Verification items for this drawing (mm, ordinates from the low corner). Round coordinates to 2 decimals unless told otherwise and drop trailing zeros. Loops run counter-clockwise (first coordinate to the right, second up) from the corner with the lowest first, then second, coordinate; pieces in that order, holes last. Notation, with made-up numbers: M 9.25,1 L 29.25,1 A25 ccw 29.25,34 Z; hole C 21,81 d4. An arc over 180 degrees is marked long. Write item = value, one per line. Start each with the question number.
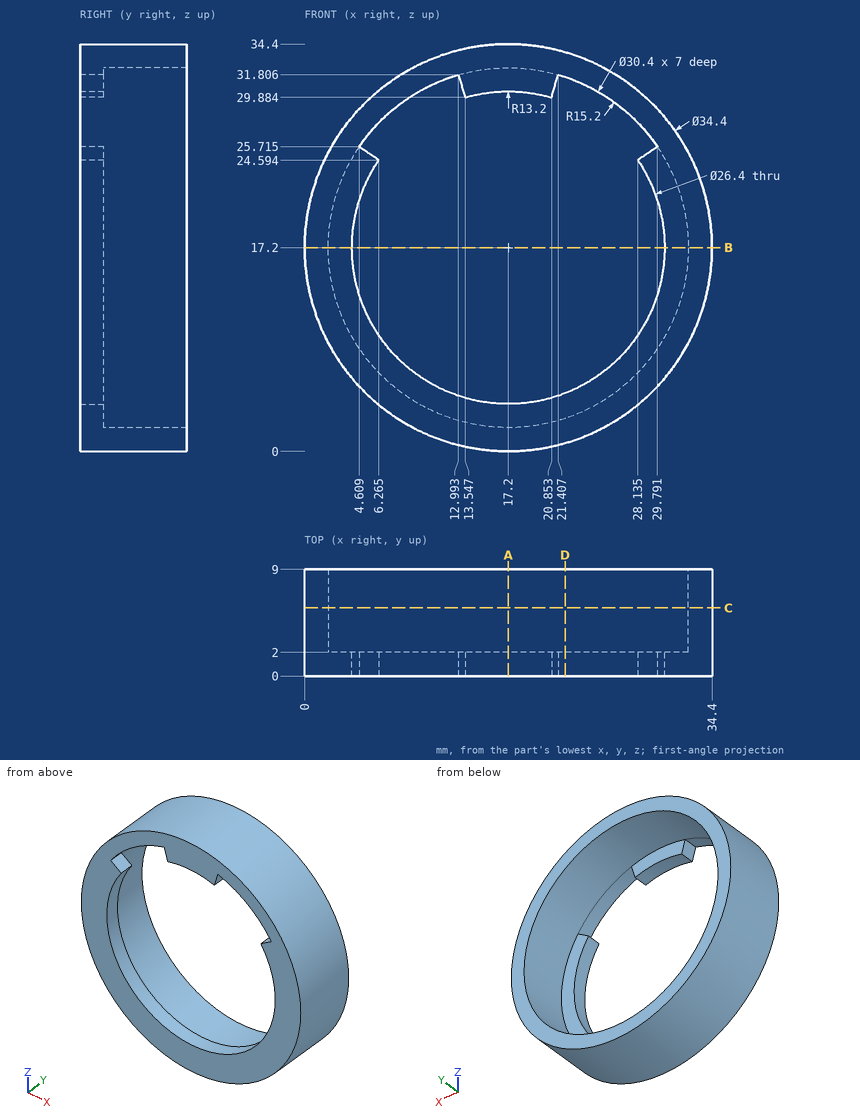
1. Gauge pin test, flat ends, axial feed: P1, Ø18, axis at x = 17.2, z = 17.2, coming from the +Y side; P2, Ø0.8, axis at x = 16, z = 31, coming from the +Y side; P3, Ø3, axis at x = 29.5, z = 12.5, coming from the -Y side; P4, Ø5, axis at y = 3.5, z = 4, coming from the +X side. Record the tip position at first contact, or that the pin passes through.
2. Thickness scan on line 1 (X direction, y = 7, z = 17.2); line 2 (Z direction, x = 17.2, y = 1.1). Record the ranges inside material, lowest first.
3. Section check C-C, the plane y = 5.75. Enter the section's corners in (x, z).
4. Section check A-A, the plane x = 17.2. Enter the section's corners in (y, z).
5. Section check D-D, the plane x = 22. Enter the section's corners in (y, z).
6. Section check B-B, the plane z = 17.2. Enter the section's corners in (x, y).
Computed values:
q1.P1 = through
q1.P2 = 2
q1.P3 = 0
q1.P4 = 30.67
q2.line_1 = 0 to 2, 32.4 to 34.4
q2.line_2 = 0 to 4, 30.4 to 34.4
q3.outline = C 17.2,17.2 d34.4; hole C 17.2,17.2 d30.4
q4.outline = M 0,0 L 9,0 L 9,2 L 2,2 L 2,4 L 0,4 Z; M 0,30.4 L 2,30.4 L 2,32.4 L 9,32.4 L 9,34.4 L 0,34.4 Z
q5.outline = M 0,0.68 L 9,0.68 L 9,2.78 L 2,2.78 L 2,4.9 L 0,4.9 Z; M 0,31.62 L 9,31.62 L 9,33.72 L 0,33.72 Z
q6.outline = M 0,0 L 4,0 L 4,2 L 2,2 L 2,9 L 0,9 Z; M 30.4,0 L 34.4,0 L 34.4,9 L 32.4,9 L 32.4,2 L 30.4,2 Z
